The drawing under review shows one solid part. Ordinate dimensions are in mm from its lowest x, y, z. A direction names the side the tool comes from. Round coordinates to 2 decimals unless told otherwise and drop trailing zeros. Order: outer loops, then holes, each group sorted by start corner. A loop starts at its lowest first (then second) coordinate and runs counter-clockwise, first axis right, second up. Notation, with made-up numbers: M 75,27.25 L 105,27.25 A14 cw 105,32.25 Z; hole C -16,46.5 d1. An arc over 180 degrees is marked long. Use a Markdown table: item, result.
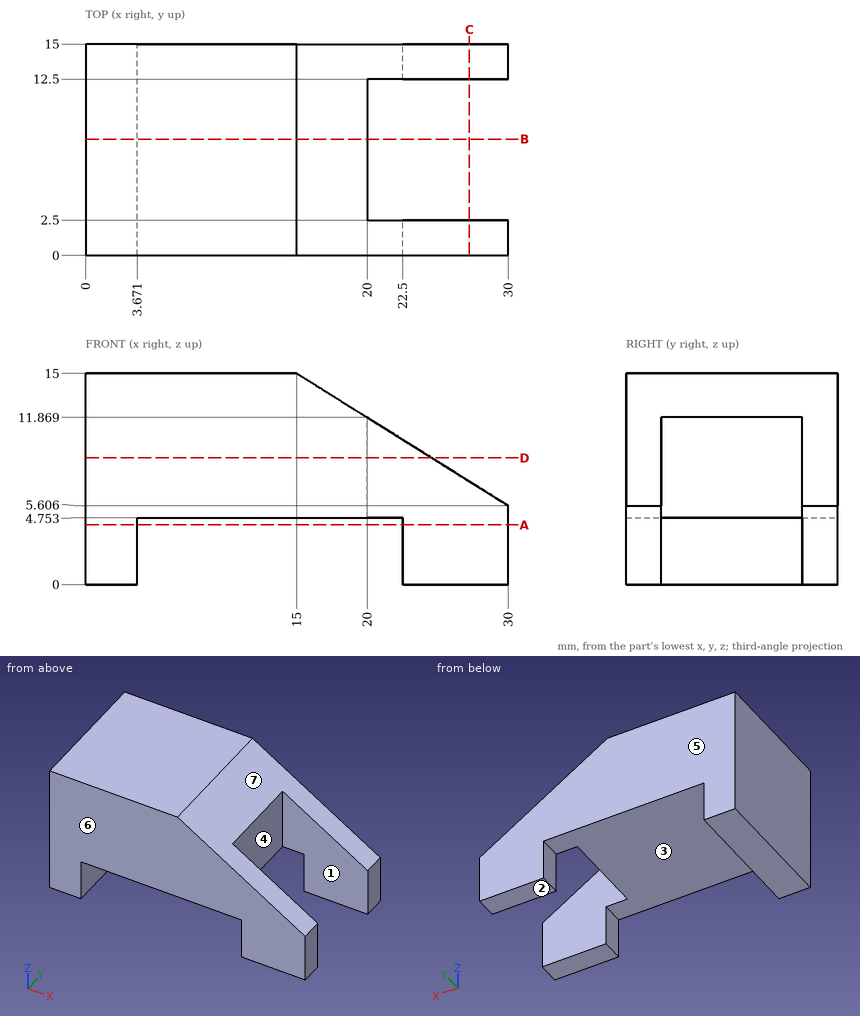
Q1. Machinability: for the marked faces 1, 2 and 3, which of the approach directions +Z, -Z, +X, -X, +Y, -Y give a long, thin tool a straight path to every point of the face, cutting with its end or side? Answer none if there is none.
Determined:
| item | result |
|---|---|
| face 1 | +Z, -Z, +X |
| face 2 | -Z, +X, -X, +Y, -Y |
| face 3 | -Z, +Y, -Y |
Q2. Wall thickness on line 1 along Y through (x, z) = (23.5, 7.5); line 2 along X through (y, z) = (1, 2.75); line 3 along Z through (x, y) = (19, 3.25) (1 decimal): over which ranges is each line inside the solid? List them lowest first. Write a range as [from, to].
Determined:
| item | result |
|---|---|
| line 1 | y = [0, 2.5], [12.5, 15] |
| line 2 | x = [0, 3.67], [22.5, 30] |
| line 3 | z = [4.8, 12.5] |
Q3. Clearance check with flat-ended pins moving along their axes: pin 1 (7.5 mm diameter, centred on x = 12, y = 9, fed in from -Z); pin 2 (2.5 mm diameter, centred on y = 5.5, z = 2, fed in from +X); pin 3 (3.5 mm diameter, centred on y = 7, z = 7, fed in from +X). State where each tip first meets the part, or that it passes through.
Determined:
| item | result |
|---|---|
| pin 1 | stops at z = 4.75 |
| pin 2 | stops at x = 3.67 |
| pin 3 | stops at x = 20 |
Q4. Add section C-C (x = 27.25). Write out the cut boundary in (y, z).
Determined:
| item | result |
|---|---|
| outline | M 0,0 L 2.5,0 L 2.5,7.33 L 0,7.33 Z; M 12.5,0 L 15,0 L 15,7.33 L 12.5,7.33 Z |
Q5. Draft analysis for pull direction Y (two halves, no side actions). For the marked faces 4, 5, 6 and 7, state which applies: pulls with the +Y half, pulls with the -Y half, needs draft (parallel to the pull), parting line crosses it, or undercut.
Determined:
| item | result |
|---|---|
| face 4 | undercut |
| face 5 | pulls with the +Y half |
| face 6 | pulls with the -Y half |
| face 7 | needs draft |
Q6. Add section D-D (z = 9). Write out the cut boundary in (x, y), then the cut area to 3 significant figures.
Determined:
| item | result |
|---|---|
| outline | M 0,0 L 24.58,0 L 24.58,2.5 L 20,2.5 L 20,12.5 L 24.58,12.5 L 24.58,15 L 0,15 Z |
| area | 323 mm^2 |
Q7. Add section A-A (z = 4.25). Write out the cut boundary in (x, y).
Determined:
| item | result |
|---|---|
| outline | M 0,0 L 3.67,0 L 3.67,15 L 0,15 Z; M 22.5,0 L 30,0 L 30,2.5 L 22.5,2.5 Z; M 22.5,12.5 L 30,12.5 L 30,15 L 22.5,15 Z |
Q8. Add section B-B (y = 8.25). Write out the cut boundary in (x, z).
Determined:
| item | result |
|---|---|
| outline | M 0,0 L 3.67,0 L 3.67,4.75 L 20,4.75 L 20,11.87 L 15,15 L 0,15 Z |
